Can you work these out from the model? Positions are in its coordinate system, mm. A direction names the side the tool comes from. Coordinates: 2 decimals unless noted, no trailing zeros. Loops run counter-clockwise (first coordinate to the right, second up) from the corner with the lowest first, then second, coordinate; pieces in that order, holes last.
```python
from build123d import *

# Parameters (mm, degrees)
BOSS_EXTRUDE1_DEPTH = 160
SKETCH2_R           = 2.5
CUT_EXTRUDE1_DEPTH  = 257.904651573
SKETCH3_W           = 54.938164949
SKETCH3_H           = 56.246543956
CUT_EXTRUDE2_DEPTH  = 257.904651573
SKETCH4_W           = 64.26610288
SKETCH4_H           = 38.441019891
CUT_EXTRUDE3_DEPTH  = 257.904651573


with BuildPart() as part:
    # Sketch1 → Boss-Extrude1 (new, symmetric)
    with BuildSketch(Plane.XY):
        Polygon((-98, 20), (-100, 20), (-100, 0), (100, 0), (100, 20), (98, 20), (98, 2), (-98, 2), align=None)
    extrude(amount=BOSS_EXTRUDE1_DEPTH, both=True)

    # Sketch2 → Cut-Extrude1 (cut, through all)
    with BuildSketch(Plane(origin=(100, 0, 0), x_dir=(0, 0, -1), z_dir=(1, 0, 0))):
        with Locations((-75.16, 10)):
            Circle(SKETCH2_R)
        with BuildLine():
            Line((-5.16, 12.5), (94.84, 12.5))
            ThreePointArc((94.84, 12.5), (97.34, 10), (94.84, 7.5))
            Line((94.84, 7.5), (-5.16, 7.5))
            ThreePointArc((-5.16, 7.5), (-7.66, 10), (-5.16, 12.5))
        make_face()
    extrude(amount=-CUT_EXTRUDE1_DEPTH, mode=Mode.SUBTRACT)

    # Sketch3 → Cut-Extrude2 (cut, through all)
    with BuildSketch(Plane(origin=(100, 0, 0), x_dir=(0, 0, -1), z_dir=(1, 0, 0))):
        with Locations((132.530917526, 28.123271978)):
            Rectangle(SKETCH3_W, SKETCH3_H)
    extrude(amount=-CUT_EXTRUDE2_DEPTH, mode=Mode.SUBTRACT)

    # Sketch4 → Cut-Extrude3 (cut, through all)
    with BuildSketch(Plane(origin=(100, 0, 0), x_dir=(0, 0, -1), z_dir=(1, 0, 0))):
        with Locations((-127.86694856, 19.220509946)):
            Rectangle(SKETCH4_W, SKETCH4_H)
    extrude(amount=-CUT_EXTRUDE3_DEPTH, mode=Mode.SUBTRACT)


solid = part.part
```
Item 1: On a 3-axis mill with a long thin cutter (end or side, diameter ignored), from which of +Z, -Z, +X, -X, +Y, -Y can I reach the whole of each face in a straight line? I mean faces 1 (the face through (-1, 0, -3)), 2 (the face through (-98, 13, -3)). Say none if no direction works.
Results are:
face 1: +Z, -Z, +X, -X, -Y
face 2: +Z, -Z, +Y
Item 2: We'd pull the mould along Y, two halves only. Please class faces 3 (the face through (-98.986, 10.751, 72.775)), 4 (the face through (1, 2, -3)), 5 (the face through (99.014, 10.751, 72.775)), 6 (the face through (0, 1, -105.062)): +Y half, -Y half, draft (parallel to the pull), parting line (faces both ways), or undercut.
Results are:
face 3: undercut
face 4: +Y half
face 5: undercut
face 6: draft
Item 3: Suppose I cut it at C-C, the plane x = -10.5. Please give me the cut outline in (y, z), plus the area to 3 significant figures.
Results are:
outline: (0, -105.06) - (2, -105.06) - (2, 95.73) - (0, 95.73) - close
area: 402 mm2
Item 4: Suppose I cut it at D-D, the plane z = 12.5. Please give me the cut outline in (x, y), plus the area to 3 significant figures.
Results are:
outline: (-100, 0) - (100, 0) - (100, 20) - (98, 20) - (98, 2) - (-98, 2) - (-98, 20) - (-100, 20) - close
area: 472 mm2
Item 5: Suppose I cut it at B-B, the plane y = 10. Please give me the cut outline in (x, z).
Results are:
outline: (-100, -105.06) - (-98, -105.06) - (-98, -97.34) - (-100, -97.34) - close; (-100, 7.66) - (-98, 7.66) - (-98, 72.66) - (-100, 72.66) - close; (-100, 77.66) - (-98, 77.66) - (-98, 95.73) - (-100, 95.73) - close; (98, -105.06) - (100, -105.06) - (100, -97.34) - (98, -97.34) - close; (98, 7.66) - (100, 7.66) - (100, 72.66) - (98, 72.66) - close; (98, 77.66) - (100, 77.66) - (100, 95.73) - (98, 95.73) - close
Item 6: Suppose I cut it at A-A, the plane z = 75.16. Please give me the cut outline in (x, y).
Results are:
outline: (-100, 0) - (100, 0) - (100, 7.5) - (98, 7.5) - (98, 2) - (-98, 2) - (-98, 7.5) - (-100, 7.5) - close; (-100, 12.5) - (-98, 12.5) - (-98, 20) - (-100, 20) - close; (98, 12.5) - (100, 12.5) - (100, 20) - (98, 20) - close
Item 7: I'm going to push flat-ended pins straight in: P1, Ø1.5, axis at x = -43.5, z = -38.5, coming from the +Y side; P2, Ø10, axis at x = 76, y = 8, coming from the -Z side. Where does each tip first touch, or does it pass through?
Results are:
P1: stops at y = 2
P2: passes through
Item 8: I need wall thicknesses on line 1 along Y through (x, z) = (-99, 75.16); line 2 along X through (y, z) = (17, 37.5); line 3 along Y through (x, z) = (-68, -28). Which ranges of each line are inside material? Lowest first, please.
Results are:
line 1: y = 0 to 7.5, 12.5 to 20
line 2: x = -100 to -98, 98 to 100
line 3: y = 0 to 2
